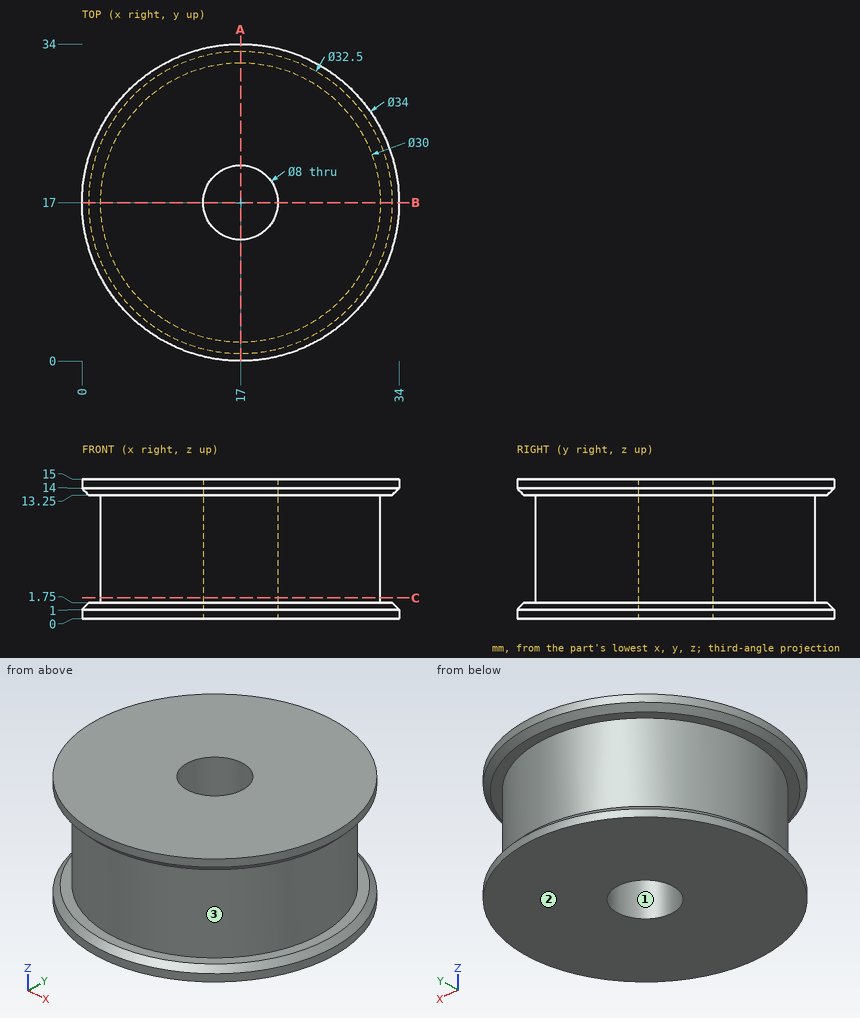
Geometry check sheet. Reference: drawing and pictorial views, mm from the part's lowest x, y, z. Round coordinates to 2 decimals unless told otherwise and drop trailing zeros. Write each loop counter-clockwise with the first axis right and the second up, starting at its lowest first coordinate (ties: lowest second). Pieces come first, ordered by that corner, then holes.
(1) Material ranges on line 1 (X direction, y = 17, z = 7.5); line 2 (Z direction, x = 26, y = 3.5); line 3 (X direction, y = 9, z = 1), recorded low to high.
Returned:
line 1: x = 2 to 13, 21 to 32
line 2: z = 0 to 1.75, 13.25 to 15
line 3: x = 2 to 32
(2) Depth check by flat-ended pin: pin 1 Ø4 at (x, z) = (22, 7) entering from -Y; pin 2 Ø3 at (y, z) = (12, 12.5) entering from +X; pin 3 Ø8 at (y, z) = (17, 9) entering from -X. Enter the tip coordinate at first touch or a pass-through.
Returned:
pin 1: stops at y = 2.3
pin 2: stops at x = 33.31
pin 3: stops at x = 2
(3) Section check C-C (z = 2.25). Enter the section's corners in (x, y), plus the area to 3 significant figures.
Returned:
outline: circle Ø30 at (17, 17); hole circle Ø8 at (17, 17)
area: 657 mm2
(4) Section check A-A (x = 17). Enter the section's corners in (y, z).
Returned:
outline: (0, 0) - (13, 0) - (13, 15) - (0, 15) - (0, 14) - (0.75, 13.25) - (2, 13.25) - (2, 1.75) - (0.75, 1.75) - (0, 1) - close; (21, 0) - (34, 0) - (34, 1) - (33.25, 1.75) - (32, 1.75) - (32, 13.25) - (33.25, 13.25) - (34, 14) - (34, 15) - (21, 15) - close
(5) Mould release check, pull along Z, two halves, no side actions. Record for the marked faces 1, 2 and 3: pulls with the +Z half, pulls with the -Z half, needs draft (parallel to the pull), parting line crosses it, or undercut.
Returned:
face 1: needs draft
face 2: pulls with the -Z half
face 3: undercut
